```python
from build123d import *

# Parameters (mm, degrees)
SKETCH_W        = 40
SKETCH_H        = 50
SKETCH_W_2      = 28
SKETCH_H_2      = 21
PAD_DEPTH       = 20
SKETCH001_R     = 2.25
POCKET_DEPTH    = 40.001
SKETCH002_W     = 29
SKETCH002_H     = 22
POCKET001_DEPTH = 19
SKETCH003_R     = 5
POCKET002_DEPTH = 5
POCKET003_DEPTH = 40.001


with BuildPart() as part:
    # Sketch → Pad (new body)
    with BuildSketch(Plane.XY):
        with Locations((20, 25)):
            Rectangle(SKETCH_W, SKETCH_H)
        with Locations((20, 25)):
            Rectangle(SKETCH_W_2, SKETCH_H_2, mode=Mode.SUBTRACT)
    extrude(amount=PAD_DEPTH)

    # Sketch001 → Pocket (cut, through all)
    with BuildSketch(Plane.YZ.offset(40)):
        with Locations((7.5, 10)):
            Circle(SKETCH001_R)
        with Locations((42.5, 10)):
            Circle(SKETCH001_R)
    extrude(amount=-POCKET_DEPTH, mode=Mode.SUBTRACT)

    # Sketch002 → Pocket001 (cut)
    with BuildSketch(Plane.XY.offset(20)):
        with Locations((20, 25)):
            Rectangle(SKETCH002_W, SKETCH002_H)
    extrude(amount=-POCKET001_DEPTH, mode=Mode.SUBTRACT)

    # Sketch003 → Pocket002 (cut)
    with BuildSketch(Plane.YZ.offset(40)):
        with Locations((7.5, 10)):
            Circle(SKETCH003_R)
        with Locations((42.5, 10)):
            Circle(SKETCH003_R)
    extrude(amount=-POCKET002_DEPTH, mode=Mode.SUBTRACT)

    # Sketch004 → Pocket003 (cut, through all)
    with BuildSketch(Plane.YZ.offset(40)):
        with BuildLine():
            ThreePointArc((17.5, 10), (14.571068, 17.071068), (7.5, 20))
            Line((7.5, 20), (7.5, 22))
            Line((7.5, 22), (42.5, 22))
            Line((42.5, 22), (42.5, 20))
            ThreePointArc((42.5, 20), (35.428932, 17.071068), (32.5, 10))
            Line((32.5, 10), (17.5, 10))
        make_face()
    extrude(amount=-POCKET003_DEPTH, mode=Mode.SUBTRACT)


solid = part.part
```
Geometry check sheet. Reference: the model listing, model coordinates, mm. A direction names the side the tool comes from. Give positions to 0.01 mm unless a question says otherwise; leave off trailing zeros. Order: outer loops, then holes, each group sorted by start corner. A loop starts at its lowest first (then second) coordinate and runs counter-clockwise, first axis right, second up. Notation, with made-up numbers: (-5, 47) - (0, 47) arc R37 ccw to (0, 86) - close; hole circle Ø2 at (11.5, 41.25). An arc over 180 degrees is marked (long way). Answer in a Markdown table with one row per item. Add a question column.
Q1. Cross-section at B-B, the plane x = 3. Enter the section's corners in (y, z).
Q2. Gauge pin test, flat ends, axial feed: pin 1 (6 mm diameter, centred on x = 2, y = 25.5, fed in from +Z); pin 2 (6 mm diameter, centred on y = 7.5, z = 10, fed in from +X). Record the tip position at first contact, or that the pin passes through.
Q3. Material ranges on probe 1 along Y at (x, z) = (13, 13); probe 2 along Z at (x, y) = (18, 42.5); probe 3 along Y at (x, z) = (21, 9), recorded low to high. Write a range as from..to.
Q4. Cross-section at C-C, the plane y = 19.5. Enter the section's corners in (x, z), then the cut area to 3 significant figures.
Q5. Mould release check, pull along Y, two halves, no side actions. Record for faces 4 (the cylindrical face through (20.28, 11.826, 19.016)), 5 (the flat face through (40, 25, 8)): pulls with the +Y half, pulls with the -Y half, needs draft (parallel to the pull), parting line crosses it, or undercut.
Q6. Cross-section at A-A, the plane x = 23. Enter the section's corners in (y, z).
Q7. Cross-section at D-D, the plane z = 3.25. Enter the section's corners in (x, y), then the cut area to 3 significant figures.
Q8. Tool access check on faces 1 (the flat face through (20, 14, 9)), 2 (the cylindrical face through (37.535, 37.505, 10.22)), 3 (the flat face through (3, 25, 10)). Record the directions out of +Z, -Z, +X, -X, +Y, -Y that give a thin tool (end or side, any length) a straight path to the whole face; none if there is none.
Check values:
| question | item | result |
|---|---|---|
| 1 | outline | (0, 0) - (50, 0) - (50, 20) - (42.5, 20) arc R10 ccw to (32.5, 10) - (17.5, 10) arc R10 ccw to (7.5, 20) - (0, 20) - close; hole circle Ø4.5 at (7.5, 10); hole circle Ø4.5 at (42.5, 10) |
| 2 | pin 1 | stops at z = 10 |
| 2 | pin 2 | stops at x = 35 |
| 3 | probe 1 | y = 0..14, 36..50 |
| 3 | probe 2 | z = 0..7.75, 12.25..20 |
| 3 | probe 3 | y = 0..5.48, 9.52..14, 36..40.48, 44.52..50 |
| 4 | outline | (0, 0) - (6, 0) - (6, 1) - (5.5, 1) - (5.5, 10) - (0, 10) - close; (34, 0) - (40, 0) - (40, 10) - (34.5, 10) - (34.5, 1) - (34, 1) - close |
| 4 | area | 111 mm^2 |
| 5 | face 4 | undercut |
| 5 | face 5 | needs draft |
| 6 | outline | (0, 0) - (14.5, 0) - (14.5, 1) - (14, 1) - (14, 17.6) arc R10 ccw to (7.5, 20) - (0, 20) - close; (35.5, 0) - (50, 0) - (50, 20) - (42.5, 20) arc R10 ccw to (36, 17.6) - (36, 1) - (35.5, 1) - close; hole circle Ø4.5 at (7.5, 10); hole circle Ø4.5 at (42.5, 10) |
| 7 | outline | (0, 0) - (40, 0) - (40, 50) - (0, 50) - close; hole (5.5, 14) - (34.5, 14) - (34.5, 36) - (5.5, 36) - close |
| 7 | area | 1,360 mm^2 |
| 8 | face 1 | +Z |
| 8 | face 2 | +X |
| 8 | face 3 | +Z, +X, -X |
